from build123d import *

# Parameters (mm, degrees)
PAD001_DEPTH           = 40
PAD_DEPTH              = 60
POCKET_DEPTH           = 425.514338
SKETCH002_W            = 5
SKETCH002_H            = 40
POCKET001_DEPTH        = 5
LINEARPATTERN_COUNT    = 11
LINEARPATTERN_PITCH    = 9.5
SKETCH003_W            = 5
SKETCH003_H            = 40
POCKET002_DEPTH        = 5
LINEARPATTERN001_COUNT = 3
LINEARPATTERN001_PITCH = 11.5
SKETCH004_W            = 5
SKETCH004_H            = 40
POCKET003_DEPTH        = 5
LINEARPATTERN002_COUNT = 3
LINEARPATTERN002_PITCH = 11.5


with BuildPart() as body001:
    # Sketch005 → Pad001 (new body)
    with BuildSketch(Plane.XY):
        Polygon((-52.93, 10), (52.93, 10), (72.93, -10), (-72.93, -10), align=None)
    extrude(amount=PAD001_DEPTH)


with BuildPart() as body001_1:
    # Body001 placement: moved
    add(body001.part.moved(Location((0, 0, 10))))


with BuildPart() as cut:
    # Sketch → Pad (new body)
    with BuildSketch(Plane.XY):
        Polygon((-55, 15), (55, 15), (85, -15), (-85, -15), align=None)
    extrude(amount=PAD_DEPTH)

    # Sketch001 (on Face6 of Pad) → Pocket (cut, through all)
    with BuildSketch(Plane.XY.offset(60)):
        Polygon((-72.928932, -10), (-52.928932, 10), (-32.928932, -10), align=None)
        Polygon((-46.465976, 10), (-26.465976, -10), (-6.465976, 10), align=None)
        Polygon((-20, -10), (0, 10), (0, -10), align=None)
    pocket = extrude(amount=-POCKET_DEPTH, mode=Mode.SUBTRACT)

    # Mirrored: Pocket across Sketch001 V_Axis
    add(pocket.mirror(Plane(origin=(0, 0, 60), x_dir=(0, 0, 1), z_dir=(1, 0, 0))), mode=Mode.SUBTRACT)

    # Sketch002 (on Face1 of Mirrored) → Pocket001 (cut)
    with BuildSketch(Plane(origin=(0, 15, 0), x_dir=(-1, 0, 0), z_dir=(0, 1, 0))):
        with Locations((-47.5, 30)):
            Rectangle(SKETCH002_W, SKETCH002_H)
    pocket001 = extrude(amount=-POCKET001_DEPTH, mode=Mode.SUBTRACT)

    # LinearPattern: Pocket001 ×11
    with Locations(*[(-i * LINEARPATTERN_PITCH, 0, 0) for i in range(1, LINEARPATTERN_COUNT)]):
        add(pocket001, mode=Mode.SUBTRACT)

    # Sketch003 (on Face5 of LinearPattern) → Pocket002 (cut)
    with BuildSketch(Plane(origin=(35, 35, 0), x_dir=(-0.707107, 0.707107, 0), z_dir=(0.707107, 0.707107, 0))):
        with Locations((-61.140678, 30)):
            Rectangle(SKETCH003_W, SKETCH003_H)
    pocket002 = extrude(amount=-POCKET002_DEPTH, mode=Mode.SUBTRACT)

    # LinearPattern001: Pocket002 ×3
    with Locations(*[Vector(-0.707107, 0.707107, 0) * (i * LINEARPATTERN001_PITCH) for i in range(1, LINEARPATTERN001_COUNT)]):
        add(pocket002, mode=Mode.SUBTRACT)

    # Sketch004 (on Face2 of LinearPattern001) → Pocket003 (cut)
    with BuildSketch(Plane(origin=(-35, 35, 0), x_dir=(-0.707107, -0.707107, 0), z_dir=(-0.707107, 0.707107, 0))):
        with Locations((61.140678, 30)):
            Rectangle(SKETCH004_W, SKETCH004_H)
    pocket003 = extrude(amount=-POCKET003_DEPTH, mode=Mode.SUBTRACT)

    # LinearPattern002: Pocket003 ×3
    with Locations(*[Vector(0.707107, 0.707107, 0) * (i * LINEARPATTERN002_PITCH) for i in range(1, LINEARPATTERN002_COUNT)]):
        add(pocket003, mode=Mode.SUBTRACT)

    # Cut: cut Body001
    add(body001_1.part, mode=Mode.SUBTRACT)


solid = cut.part
Here's how the part is built. I have some questions about the finished solid (model axes, mm). A direction names the side the tool comes from. Round coordinates to 2 decimals unless told otherwise and drop trailing zeros. Loops run counter-clockwise (first coordinate to the right, second up) from the corner with the lowest first, then second, coordinate; pieces in that order, holes last. Notation, with made-up numbers: M -38,32.5 L 16,32.5 A22 ccw 16,57.5 Z; hole C 32,8.5 d3. An arc over 180 degrees is marked long. Write each question's results on one line, items separated by ' | '. Start each with the question number.
(1) Will these pins go through, and if not, where does the flat tip stop? P1, Ø12, axis at y = -3.5, z = 28, coming from the +X side; P2, Ø1.5, axis at y = -2.5, z = 19.5, coming from the -X side; P3, Ø2.5, axis at y = 11.5, z = 39.5, coming from the +X side.
(2) I want a section at A-A (z = 56). Please give me the cut outline in (x, y).
(3) I want a section at C-C (y = 11.5). State how many separate pieces and enclosed holes the cut face has, then the cut area to 3 significant figures.
(4) On a 3-axis mill with a long thin cutter (end or side, diameter ignored), from which of +Z, -Z, +X, -X, +Y, -Y can I reach the whole of each face in a straight line? I mean faces 1 (the flat face through (4, 7, 10)), 2 (the flat face through (7, 13, 30)), 3 (the flat face through (-43.07, 0.14, 55.07)). Say none if no direction works.
(5) I want a section at B-B (x = 24.5). Please give me the cut outline in (y, z).
(6) Thinking about a two-plate mould opening in Z: for faces 4 (the flat face through (-43.07, 0.14, 5.07)), 5 (the flat face through (-26, 13, 30)), which applies, pulls with the +Z half, pulls with the -Z half, needs draft (parallel to the pull), parting line crosses it, or undercut?
(7) If I drill on probe 1 along Z at (x, y) = (47.5, 14.5); probe 2 along X at (y, z) = (-8, 7); probe 3 along X at (y, z) = (-1, 53), over which ranges is the centre line in solid material (lowest first)? Write a range as from..to.
Solved:
1) P1: stops at x = 76.47 | P2: stops at x = -73.25 | P3: stops at x = 59.75
2) outline: M -85,-15 L 85,-15 L 55,15 L -55,15 Z; hole M -72.93,-10 L -32.93,-10 L -52.93,10 Z; hole M -46.47,10 L -26.47,-10 L -6.47,10 Z; hole M -20,-10 L 20,-10 L 0,10 Z; hole M 6.47,10 L 26.47,-10 L 46.47,10 Z; hole M 32.93,-10 L 72.93,-10 L 52.93,10 Z
3) separate pieces: 1 | enclosed holes: 11 | area: 4,820 mm²
4) face 1: none | face 2: +Y | face 3: +Z, -Z
5) outline: M -15,0 L -8.03,0 L -8.03,10 L -10,10 L -10,50 L -8.03,50 L -8.03,60 L -15,60 Z; M 10,0 L 15,0 L 15,60 L 10,60 Z
6) face 4: needs draft | face 5: undercut
7) probe 1: z = 0..10, 50..60 | probe 2: x = -78..-70.93, -34.93..-28.47, -24.47..-18, 18..24.47, 28.47..34.93, 70.93..78 | probe 3: x = -71..-63.93, -41.93..-35.47, -17.47..-11, 11..17.47, 35.47..41.93, 63.93..71
